Answer from the drawing. Dimensions are ordinates in mm from the lowest x, y and z of the part. A direction names the side the tool comes from. Coordinates: 2 decimals unless noted, no trailing zeros. Loops run counter-clockwise (first coordinate to the right, second up) from the corner with the lowest first, then second, coordinate; pieces in that order, holes last. Notation, with made-up numbers: (57.25, 63.5) - (110.25, 63.5) arc R31 cw to (110.25, 91.5) - close; hole circle Ø10 at (36.5, 36). An arc over 180 degrees is marked (long way). Write each question's results on one line, items separated by ' | '. Start each with the question number.
1. Determine the mould class of the marked faces 4, 5 and 6 for opening direction X: released by +X, released by -X, zero draft, split by the parting line, or undercut.
2. A cutting plane is placed at D-D on y = 5. Determine the outline of the cut face in (x, z), then the cut area to 3 significant figures.
3. Which of the six approach directions +Z, -Z, +X, -X, +Y, -Y give full straight-line access (tool end or side, diameter ignored) to the marked faces 1, 2 and 3?
4. A cutting plane is placed at C-C on z = 3.4. Determine the outline of the cut face in (x, y) (3 decimals), then the cut area to 3 significant figures.
5. A cutting plane is placed at B-B on x = 27. Determine the outline of the cut face in (y, z).
6. Each of these flat-tipped pins is pushed along its axis until it touches: P1, Ø1.8, axis at x = 47, z = 1.5, coming from the -Y side; P2, Ø3, axis at y = 8.5, z = 3.5, coming from the +X side. Where does it stop, or does it pass through?
7. Find the intervals of material crossed by line 1 along Y through (x, z) = (12.5, 2.1); line 2 along X through (y, z) = (16.5, 3.45); line 3 along Y through (x, z) = (3, 4.95), in increasing order. Write a range as [from, to].
8. A cutting plane is placed at A-A on y = 34.75. Determine the outline of the cut face in (x, z) (3 decimals).
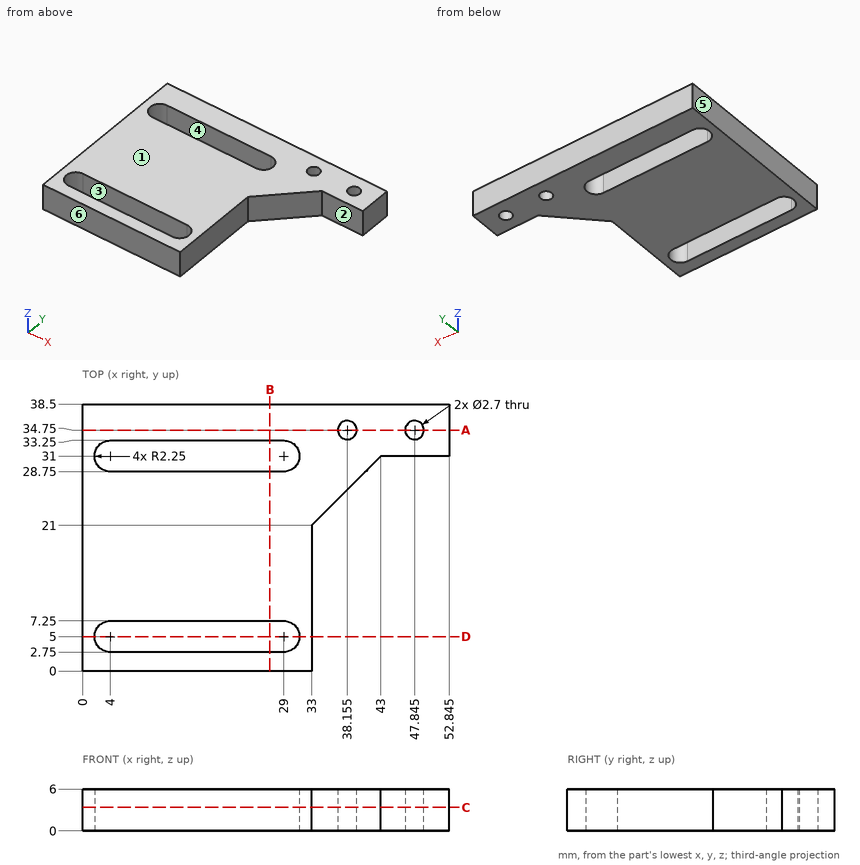
Values:
1) face 4: undercut | face 5: released by -X | face 6: zero draft
2) outline: (0, 0) - (1.75, 0) - (1.75, 6) - (0, 6) - close; (31.25, 0) - (33, 0) - (33, 6) - (31.25, 6) - close | area: 21.0 mm^2
3) face 1: +Z, +X, -X, +Y, -Y | face 2: +Z, -Z, +X, -Y | face 3: +Z, -Z
4) outline: (0, 0) - (33, 0) - (33, 21) - (43, 31) - (52.845, 31) - (52.845, 38.5) - (0, 38.5) - close; hole (4, 2.75) - (29, 2.75) arc R2.25 ccw to (29, 7.25) - (4, 7.25) arc R2.25 ccw to start; hole (4, 28.75) - (29, 28.75) arc R2.25 ccw to (29, 33.25) - (4, 33.25) arc R2.25 ccw to start; hole circle Ø2.7 at (38.155, 34.75); hole circle Ø2.7 at (47.845, 34.75) | area: 1,200 mm^2
5) outline: (0, 0) - (2.75, 0) - (2.75, 6) - (0, 6) - close; (7.25, 0) - (28.75, 0) - (28.75, 6) - (7.25, 6) - close; (33.25, 0) - (38.5, 0) - (38.5, 6) - (33.25, 6) - close
6) P1: y = 31 | P2: x = 33
7) line 1: [0, 2.75], [7.25, 28.75], [33.25, 38.5] | line 2: [0, 33] | line 3: [0, 2.98], [7.02, 28.98], [33.02, 38.5]
8) outline: (0, 0) - (36.805, 0) - (36.805, 6) - (0, 6) - close; (39.505, 0) - (46.495, 0) - (46.495, 6) - (39.505, 6) - close; (49.195, 0) - (52.845, 0) - (52.845, 6) - (49.195, 6) - close
